Input: part model. Units: mm. Frame: model coordinates. A direction names the side the tool comes from. Coordinates: 2 decimals unless noted, no trailing zeros. Loops run counter-clockwise (first coordinate to the right, second up) from the corner with the lowest first, then second, coordinate; pieces in that order, holes last. Notation, with made-up numbers: (43, -31.75) - (65, -31.75) arc R23 ccw to (65, -8.75) - close; hole circle Ø11 at (38.5, 33). An arc over 180 degrees is marked (long way). Use a Markdown table: item, result. Add a question column.
1. Draft query along Y for faces 3 (the face through (-78.495, -0.434, 1.972)), 4 (the face through (58, 0, 2)), 5 (the face through (-21, 0, 4)), 6 (the face through (2.107, -12.096, 1.972)). Return one class per face: released by +Y, released by -Y, zero draft, split by the parting line, or undercut.
2. Contact query for flat-ended pins moving along their axis: P1, Ø1.5, axis at x = -36.5, z = 2.5, coming from the -Y side; P2, Ø0.8, axis at y = -10.5, z = 1, coming from the -X side; P3, Ø0.5, axis at y = 10.5, z = 2.5, coming from the -X side; P4, Ø5, axis at x = -60, y = 0, coming from the -Z side. Output: stop coordinate, or through.
3. Section query A-A on y = 0. Return the cut outline in (x, z).
4. Section query C-C on z = 3.1. Return the cut outline in (x, y) (3 decimals).
5. Section query B-B on x = -60. Return the cut outline in (y, z), then the cut area to 3 significant figures.
6. Ray query, L1, parallel to Y at x = -60, z = 1.3; L2, parallel to X at y = -2.5, z = 2.8; L3, parallel to X at y = 0.5, z = 1.25. Return the intervals inside material, ascending. Write a range as [from, to].
7. Access query for faces 1 (the face through (-21, 0, 0)), 2 (the face through (-60, -8.5, 2)). Directions: +Z, -Z, +X, -X, +Y, -Y. A direction counts if a zero-diameter tool reaches every point of the face in a straight line with its end or side. Return the directions, or none.
8. Section query D-D on x = -45. Return the cut outline in (y, z).
```python
from build123d import *

# Parameters (mm, degrees)
SKETCH1_R           = 2
SKETCH1_R_2         = 4
BOSS_EXTRUDE1_DEPTH = 4


with BuildPart() as part:
    # Sketch1 → Boss-Extrude1 (new body)
    with BuildSketch(Plane.XY):
        with BuildLine():
            Line((-58.072916667, 18.399357321), (60.625, 5.967359131))
            ThreePointArc((60.625, 5.967359131), (66, 0), (60.625, -5.967359131))
            Line((60.625, -5.967359131), (-58.072916667, -18.399357321))
            ThreePointArc((-58.072916667, -18.399357321), (-78.5, 0), (-58.072916667, 18.399357321))
        make_face()
        with Locations((60, 0)):
            Circle(SKETCH1_R, mode=Mode.SUBTRACT)
        with Locations((-60, 0)):
            Circle(SKETCH1_R_2, mode=Mode.SUBTRACT)
        with BuildLine():
            Line((-58.5, 11), (-58.5, 10))
            ThreePointArc((-58.5, 10), (-60, 8.5), (-61.5, 10))
            Line((-61.5, 10), (-61.5, 11))
            ThreePointArc((-61.5, 11), (-60, 12.5), (-58.5, 11))
        make_face(mode=Mode.SUBTRACT)
        with BuildLine():
            Line((-58.5, -11), (-58.5, -10))
            ThreePointArc((-58.5, -10), (-60, -8.5), (-61.5, -10))
            Line((-61.5, -10), (-61.5, -11))
            ThreePointArc((-61.5, -11), (-60, -12.5), (-58.5, -11))
        make_face(mode=Mode.SUBTRACT)
    extrude(amount=BOSS_EXTRUDE1_DEPTH)


solid = part.part
```
Resolved:
| question | item | result |
|---|---|---|
| 1 | face 3 | split by the parting line |
| 1 | face 4 | undercut |
| 1 | face 5 | zero draft |
| 1 | face 6 | released by -Y |
| 2 | P1 | y = -16.22 |
| 2 | P2 | x = -75.5 |
| 2 | P3 | x = -75.4 |
| 2 | P4 | through |
| 3 | outline | (-78.5, 0) - (-64, 0) - (-64, 4) - (-78.5, 4) - close; (-56, 0) - (58, 0) - (58, 4) - (-56, 4) - close; (62, 0) - (66, 0) - (66, 4) - (62, 4) - close |
| 4 | outline | (-58.073, -18.399) - (60.625, -5.967) arc R6 ccw to (60.625, 5.967) - (-58.073, 18.399) arc R18.5 ccw (long way) to start; hole circle Ø8 at (-60, 0); hole (-61.5, -11) arc R1.5 ccw to (-58.5, -11) - (-58.5, -10) arc R1.5 ccw to (-61.5, -10) - close; hole (-61.5, 10) arc R1.5 ccw to (-58.5, 10) - (-58.5, 11) arc R1.5 ccw to (-61.5, 11) - close; hole circle Ø4 at (60, 0) |
| 5 | outline | (-18.5, 0) - (-12.5, 0) - (-12.5, 4) - (-18.5, 4) - close; (-8.5, 0) - (-4, 0) - (-4, 4) - (-8.5, 4) - close; (4, 0) - (8.5, 0) - (8.5, 4) - (4, 4) - close; (12.5, 0) - (18.5, 0) - (18.5, 4) - (12.5, 4) - close |
| 5 | area | 84.0 mm² |
| 6 | L1 | [-18.5, -12.5], [-8.5, -4], [4, 8.5], [12.5, 18.5] |
| 6 | L2 | [-78.33, -63.12], [-56.88, 65.45] |
| 6 | L3 | [-78.49, -63.97], [-56.03, 58.06], [61.94, 65.98] |
| 7 | face 1 | -Z, +X, -X, +Y, -Y |
| 7 | face 2 | +Z, -Z |
| 8 | outline | (-17.03, 0) - (17.03, 0) - (17.03, 4) - (-17.03, 4) - close |
